```python
from build123d import *

# Parameters (mm, degrees)
SKETCH_1_R           = 1.25
EXTRUDE_1_DEPTH      = 3
SKETCH_2_R           = 1.5
CUT_EXTRUDE_1_DEPTH  = 3
CUT_EXTRUDE_2_DEPTH  = 3
CUT_EXTRUDE_3_DEPTH  = 3
CUT_EXTRUDE_4_DEPTH  = 10
SKETCH_6_R           = 1.5
CUT_EXTRUDE_5_DEPTH  = 10
SKETCH_7_R           = 1.5
CUT_EXTRUDE_8_DEPTH  = 10
SKETCH_8_R           = 1.5
CUT_EXTRUDE_9_DEPTH  = 10
SKETCH_9_R           = 15
CUT_EXTRUDE_10_DEPTH = 10


with BuildPart() as part:
    # 草图1 → 凸台-拉伸1 (new body)
    # profile 1 of 4: a face of its own
    with BuildSketch(Plane(origin=(0, 0, 0), x_dir=(1, 0, 0), z_dir=(0, 1, 0))):
        with BuildLine():
            ThreePointArc((75, -15), (32.573593129, -32.573593129), (15, -75))
            Line((15, -75), (0, -75))
            Line((0, -75), (0, 0))
            Line((0, 0), (75, 0))
            Line((75, 0), (75, -15))
        make_face()
        with Locations(Location((11, -70, 0), (0, 0, 270))):
            Circle(SKETCH_1_R, mode=Mode.SUBTRACT)
        with Locations(Location((70, -11, 0), (0, 0, 270))):
            Circle(SKETCH_1_R, mode=Mode.SUBTRACT)
    # profile 2 of 4: a face of its own
    with BuildSketch(Plane(origin=(0, 0, 0), x_dir=(1, 0, 0), z_dir=(0, 1, 0))):
        with BuildLine():
            ThreePointArc((-15, -75), (-32.573593129, -32.573593129), (-75, -15))
            Line((-75, -15), (-75, 0))
            Line((-75, 0), (0, 0))
            Line((0, 0), (0, -75))
            Line((0, -75), (-15, -75))
        make_face()
        with Locations(Location((-70, -11, 0), (0, 0, 270))):
            Circle(SKETCH_1_R, mode=Mode.SUBTRACT)
        with Locations(Location((-11, -70, 0), (0, 0, 270))):
            Circle(SKETCH_1_R, mode=Mode.SUBTRACT)
    # profile 3 of 4: a face of its own
    with BuildSketch(Plane(origin=(0, 0, 0), x_dir=(1, 0, 0), z_dir=(0, 1, 0))):
        with BuildLine():
            ThreePointArc((-75, 15), (-32.573593129, 32.573593129), (-15, 75))
            Line((-15, 75), (0, 75))
            Line((0, 75), (0, 0))
            Line((0, 0), (-75, 0))
            Line((-75, 0), (-75, 15))
        make_face()
        with Locations(Location((-11, 70, 0), (0, 0, 270))):
            Circle(SKETCH_1_R, mode=Mode.SUBTRACT)
        with Locations(Location((-70, 11, 0), (0, 0, 270))):
            Circle(SKETCH_1_R, mode=Mode.SUBTRACT)
    # profile 4 of 4: a face of its own
    with BuildSketch(Plane(origin=(0, 0, 0), x_dir=(1, 0, 0), z_dir=(0, 1, 0))):
        with BuildLine():
            ThreePointArc((15, 75), (32.573593129, 32.573593129), (75, 15))
            Line((75, 15), (75, 0))
            Line((75, 0), (0, 0))
            Line((0, 0), (0, 75))
            Line((0, 75), (15, 75))
        make_face()
        with Locations(Location((70, 11, 0), (0, 0, 270))):
            Circle(SKETCH_1_R, mode=Mode.SUBTRACT)
        with Locations(Location((11, 70, 0), (0, 0, 270))):
            Circle(SKETCH_1_R, mode=Mode.SUBTRACT)
    extrude(amount=EXTRUDE_1_DEPTH)

    # 草图2 → 切除-拉伸1 (cut)
    with BuildSketch(Plane.XZ):
        with Locations(Location((0.353553391, -31.466251763, 0), (0, 0, 270))):
            Circle(SKETCH_2_R)
        with Locations(Location((31.466251763, -0.353553391, 0), (0, 0, 270))):
            Circle(SKETCH_2_R)
        with Locations(Location((-0.353553391, 31.466251763, 0), (0, 0, 90))):
            Circle(SKETCH_2_R)
        with Locations(Location((-31.466251763, 0.353553391, 0), (0, 0, 90))):
            Circle(SKETCH_2_R)
    extrude(amount=-CUT_EXTRUDE_1_DEPTH, mode=Mode.SUBTRACT)

    # 草图3 → 切除-拉伸2 (cut)
    with BuildSketch(Plane(origin=(0, 3, 0), x_dir=(1, 0, 0), z_dir=(0, 1, 0))):
        Polygon((-15.556349186, 15.556349186), (-12.02081528, 19.091883092), (-22.627416998, 22.627416998), align=None)
        Polygon((-19.091883092, 12.02081528), (-15.556349186, 15.556349186), (-22.627416998, 22.627416998), align=None)
    extrude(amount=-CUT_EXTRUDE_2_DEPTH, mode=Mode.SUBTRACT)

    # 草图4 → 切除-拉伸3 (cut)
    with BuildSketch(Plane(origin=(0, 3, 0), x_dir=(1, 0, 0), z_dir=(0, 1, 0))):
        with BuildLine():
            ThreePointArc((33.944668714, -19.80253309), (34.043922781, -8.582763971), (22.827665534, -8.285032838))
            Line((22.827665534, -8.285032838), (15.556349186, -15.556349186))
            Line((15.556349186, -15.556349186), (8.285032838, -22.827665534))
            ThreePointArc((8.285032838, -22.827665534), (8.582763971, -34.043922781), (19.80253309, -33.944668714))
            Line((19.80253309, -33.944668714), (33.944668714, -19.80253309))
        make_face()
    extrude(amount=-CUT_EXTRUDE_3_DEPTH, mode=Mode.SUBTRACT)

    # 草图5 → 切除-拉伸4 (cut)
    with BuildSketch(Plane(origin=(0, 3, 0), x_dir=(1, 0, 0), z_dir=(0, 1, 0))):
        Polygon((-22.627416998, 8.485281374), (-22.627416998, 22.627416998), (-19.091883092, 12.02081528), align=None)
        Polygon((-12.02081528, 19.091883092), (-22.627416998, 22.627416998), (-8.485281374, 22.627416998), align=None)
    extrude(amount=-CUT_EXTRUDE_4_DEPTH, mode=Mode.SUBTRACT)

    # 草图6 → 切除-拉伸5 (cut)
    with BuildSketch(Plane(origin=(0, 3, 0), x_dir=(1, 0, 0), z_dir=(0, 1, 0))):
        with Locations(Location((-35.355339059, -21.213203436, 0), (0, 0, 270))):
            Circle(SKETCH_6_R)
        with Locations(Location((-21.213203436, -35.355339059, 0), (0, 0, 270))):
            Circle(SKETCH_6_R)
        with Locations(Location((35.355339059, 21.213203436, 0), (0, 0, 270))):
            Circle(SKETCH_6_R)
        with Locations(Location((21.213203436, 35.355339059, 0), (0, 0, 270))):
            Circle(SKETCH_6_R)
    extrude(amount=-CUT_EXTRUDE_5_DEPTH, mode=Mode.SUBTRACT)

    # 草图7 → 切除-拉伸8 (cut)
    with BuildSketch(Plane(origin=(0, 3, 0), x_dir=(1, 0, 0), z_dir=(0, 1, 0))):
        with Locations(Location((-29.69848481, 29.69848481, 0), (0, 0, 270))):
            Circle(SKETCH_7_R)
        with Locations(Location((29.69848481, 29.69848481, 0), (0, 0, 270))):
            Circle(SKETCH_7_R)
        with Locations(Location((29.69848481, -29.69848481, 0), (0, 0, 270))):
            Circle(SKETCH_7_R)
        with Locations(Location((-29.69848481, -29.69848481, 0), (0, 0, 270))):
            Circle(SKETCH_7_R)
    extrude(amount=-CUT_EXTRUDE_8_DEPTH, mode=Mode.SUBTRACT)

    # 草图8 → 切除-拉伸9 (cut)
    with BuildSketch(Plane(origin=(0, 3, 0), x_dir=(1, 0, 0), z_dir=(0, 1, 0))):
        with Locations(Location((-11, 55, 0), (0, 0, 270))):
            Circle(SKETCH_8_R)
        with Locations(Location((11, 55, 0), (0, 0, 270))):
            Circle(SKETCH_8_R)
        with Locations(Location((55, 11, 0), (0, 0, 270))):
            Circle(SKETCH_8_R)
        with Locations(Location((55, -11, 0), (0, 0, 270))):
            Circle(SKETCH_8_R)
        with Locations(Location((11, -55, 0), (0, 0, 270))):
            Circle(SKETCH_8_R)
        with Locations(Location((-11, -55, 0), (0, 0, 270))):
            Circle(SKETCH_8_R)
        with Locations(Location((-55, -11, 0), (0, 0, 270))):
            Circle(SKETCH_8_R)
        with Locations(Location((-55, 11, 0), (0, 0, 270))):
            Circle(SKETCH_8_R)
    extrude(amount=-CUT_EXTRUDE_9_DEPTH, mode=Mode.SUBTRACT)

    # 草图9 → 切除-拉伸10 (cut)
    with BuildSketch(Plane(origin=(0, 3, 0), x_dir=(1, 0, 0), z_dir=(0, 1, 0))):
        with Locations(Location((0, 0, 0), (0, 0, 270))):
            Circle(SKETCH_9_R)
    extrude(amount=-CUT_EXTRUDE_10_DEPTH, mode=Mode.SUBTRACT)


solid = part.part
```
Verification items for the finished model (mm, model axes). A direction names the side the tool comes from. Give positions to 0.01 mm unless a question says otherwise; leave off trailing zeros. Order: outer loops, then holes, each group sorted by start corner. A loop starts at its lowest first (then second) coordinate and runs counter-clockwise, first axis right, second up. Notation, with made-up numbers: (17.25, 70) - (44.25, 70) arc R22 ccw to (44.25, 76) - close; hole circle Ø9 at (31, 31). An arc over 180 degrees is marked (long way). Answer as CSV lines item,"result". Start each with the question number.
Item 1: Section check D-D, the plane z = 39. Record the boundary of the cut face in (x, y).
Item 2: Mould release check, pull along Z, two halves, no side actions. Record for faces 1 (the face through (-16, 3, -1)), 2 (the face through (32.11, 1.48, -33.04)), 3 (the face through (8.459, 1.521, 33.922)): released by +Z, released by -Z, zero draft, split by the parting line, or undercut.
Item 3: Section check A-A, the plane z = -17.5. Record the boundary of the cut face in (x, y).
Item 4: Gauge pin test, flat ends, axial feed: pin 1 (5 mm diameter, centred on x = -21.21, z = 35.36, fed in from +Y); pin 2 (1 mm diameter, centred on x = -57.5, y = 2, fed in from -Z); pin 3 (2.5 mm diameter, centred on x = 35.36, z = -21.21, fed in from +Y). Record the tip position at first contact, or that the pin passes through.
Item 5: Section check C-C, the plane x = 43.5. Record the boundary of the cut face in (y, z), plus the area to 3 significant figures.
Item 6: Access from +Z, -Z, +X, -X, +Y, -Y to the whole of each face (thin tool, end or side, straight path). Record for faces 4 (the face through (-15.457, 1.521, -15.655)), 5 (the face through (-33.04, 1.48, -32.11)).
Item 7: Section check B-B, the plane y = 2.35. State how many separate pieces and enclosed holes the cut face has, plus the area to 3 significant figures.
Item 8: Material ranges on L1, parallel to Z at x = -0.5, y = 1.9; L2, parallel to Z at x = 20, y = 0.5; L3, parallel to Z at x = 69.5, y = 1.2, recorded low to high.
Filled in:
1,outline,"(-27, 0) - (27, 0) - (27, 3) - (-27, 3) - close"
2,face 1,"zero draft"
2,face 2,"released by -Z"
2,face 3,"undercut"
3,outline,"(-57.86, 0) - (-22.63, 0) - (-22.63, 3) - (-57.86, 3) - close; (-13.61, 0) - (57.86, 0) - (57.86, 3) - (-13.61, 3) - close"
4,pin 1,"y = 3"
4,pin 2,"z = -17.76"
4,pin 3,"through"
5,outline,"(0, -23.93) - (3, -23.93) - (3, 23.93) - (0, 23.93) - close"
5,area,"144 mm^2"
6,face 4,"+Y, -Y"
6,face 5,"-Z, -X, +Y, -Y"
7,separate pieces,"1"
7,enclosed holes,"31"
7,area,"9,680 mm^2"
8,L1,"-75 to -32.7, -30.23 to -14.99, 14.99 to 29.97, 32.96 to 75"
8,L2,"-51.02 to -36.24, -34.47 to 11.11, 33.75 to 51.02"
8,L3,"-15.25 to -12.15, -9.85 to 9.85, 12.15 to 15.25"
